Autodesk Inventor part; units mm, degrees
ref_plane "Work Plane2" through (0, 0, 5) normal (0, 0, 1) x (1, 0, 0)
ref_plane "Work Plane8" through (0, 0, 0) normal (0.9238795, 0.3826834, 0) x (0, 0, 1)
ref_plane "Work Plane9" through (0, 0, 0) normal (1, 0, 0) x (0, 1, 0)
sketch "Sketch1" plane through (0, 0, 0) normal (0, 0, 1) x (1, 0, 0)
  circle A0 centre (0, 0) radius 5
  dimension "d0" = 10
extrude "Extrusion1" add sketch "Sketch1" along normal blind 10
ref_plane "Work Plane2" through (0, 0, 5) normal (0, 0, 1) x (1, 0, 0)
sketch "Sketch2" plane through (0, 0, 0) normal (0, 0, -1) x (-1, 0, 0)
  circle A0 centre (0, 0) radius 5
  circle A1 centre (0, 0) radius 4
  dimension "d3" = 8
surface extrude "Pitch Diameter" sketch "Sketch2" against normal through all shown no curves A1
ref_plane "Work Plane8" through (0, 0, 0) normal (0.9238795, 0.3826834, 0) x (0, 0, 1)
ref_plane "Work Plane9" through (0, 0, 0) normal (1, 0, 0) x (0, 1, 0)
spur gear teeth "Spur Gear" teeth 8 pitch diameter 8 tip diameter 10 root diameter 5.5 face width 10 start plane through (0, 0, 0) normal (0, 0, -1) x (-1, 0, 0)
equation "\"d0\" = da_da"
equation "\"d1\" = da_b"
equation "\"d3\" = da_d"
equation "\"d16\" = da_aw"
equation "\"d43\" = da_aw"
equation "\"d46\" = da_aw"
properties part number "Spur Gear1" material "Steel"
Design review of the part built by this model. Coordinates are the model's own, in mm. A direction names the side the tool comes from. Give positions to 0.01 mm unless a question says otherwise; leave off trailing zeros. Write each loop counter-clockwise with the first axis right and the second up, starting at its lowest first coordinate (ties: lowest second). Pieces come first, ordered by that corner, then holes. Notation, with made-up numbers: M -0.5,73.25 L 3.5,73.25 A20 cw 3.5,78.25 Z; hole C 87.5,17 d3. An arc over 180 degrees is marked long. Answer as a JSON object with one key per item and string values. Group by question number.
1) We need section B-B (y = -3.5). Give the boundary of the cut face in (x, z), and give its area (3 significant figures).
2) Tool access review of faces 1 (the face through (-3.255, 2.129, 4.93)), 2 (the face through (-0.797, 3.807, 4.93)), 3 (the face through (-2.129, -3.255, 4.93)): name each direction out of +Z, -Z, +X, -X, +Y, -Y from which nothing blocks a thin tool from reaching the whole face with its end or side.
3) We need section D-D (x = -1.5). Give the boundary of the cut face in (y, z), and give its area (3 significant figures).
4) Mouldability with a two-part tool opening along Y and no side actions: class faces 4 (the face through (0, -5, 5)), 5 (the face through (5, 0, 5)), 6 (the face through (3.255, -2.129, 4.93)) as released by +Y, released by -Y, zero draft, split by the parting line, or undercut.
5) For line 1 along X through (y, z) = (2.5, 5.5); line 2 along Y through (x, z) = (3.25, 7.5), list the stretches that pass through material, from the lowest coordinate up.
Answer key:
{
 "1": {"outline": "M -3.57,0 L -2.48,0 L -2.48,10 L -3.57,10 Z; M -0.83,0 L 0.83,0 L 0.83,10 L -0.83,10 Z; M 2.48,0 L 3.57,0 L 3.57,10 L 2.48,10 Z", "area": "38.4 mm²"},
 "2": {"face 1": "+Z, -Z, -X", "face 2": "+Z, -Z", "face 3": "+Z, -Z, -Y"},
 "3": {"outline": "M -2.67,0 L 2.67,0 L 2.67,10 L -2.67,10 Z", "area": "53.4 mm²"},
 "4": {"face 4": "released by -Y", "face 5": "split by the parting line", "face 6": "undercut"},
 "5": {"line 1": "x = -3.51 to -1.36, -1.15 to 1.15, 1.36 to 3.51", "line 2": "y = -3.8 to -2.12, -0.83 to 0.83, 2.12 to 3.8"}
}
